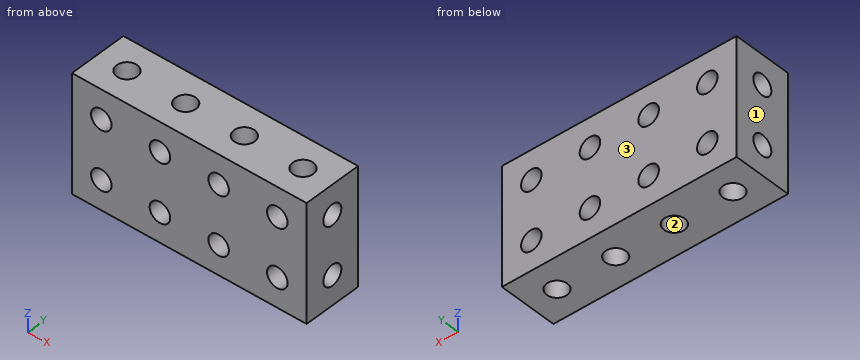
from build123d import *

# Parameters (mm, degrees)
ESQUISSE1_W             = 20
ESQUISSE1_H             = 10
BOSS_EXTRU_1_DEPTH      = 40
ESQUISSE2_R             = 1.75
ENL_V_MAT_EXTRU_1_DEPTH = 46.82575695
ESQUISSE3_R             = 1.75
ENL_V_MAT_EXTRU_2_DEPTH = 40
ESQUISSE4_R             = 1.75
ENL_V_MAT_EXTRU_3_DEPTH = 40


with BuildPart() as part:
    # Esquisse1 → Boss.-Extru.1 (new body)
    with BuildSketch(Plane(origin=(0, 0, 0), x_dir=(0, 0, -1), z_dir=(1, 0, 0))):
        with Locations((10, 5)):
            Rectangle(ESQUISSE1_W, ESQUISSE1_H)
    extrude(amount=BOSS_EXTRU_1_DEPTH)

    # Esquisse2 → Enlèv. mat.-Extru.1 (cut, through all)
    with BuildSketch(Plane(origin=(0, 10, 0), x_dir=(1, 0, 0), z_dir=(0, 1, 0))):
        with Locations(Location((5, 15, 0), (0, 0, 270))):
            Circle(ESQUISSE2_R)
        with Locations(Location((15, 15, 0), (0, 0, 270))):
            Circle(ESQUISSE2_R)
        with Locations(Location((25, 15, 0), (0, 0, 270))):
            Circle(ESQUISSE2_R)
        with Locations(Location((35, 15, 0), (0, 0, 270))):
            Circle(ESQUISSE2_R)
        with Locations(Location((5, 5, 0), (0, 0, 270))):
            Circle(ESQUISSE2_R)
        with Locations(Location((15, 5, 0), (0, 0, 270))):
            Circle(ESQUISSE2_R)
        with Locations(Location((25, 5, 0), (0, 0, 270))):
            Circle(ESQUISSE2_R)
        with Locations(Location((35, 5, 0), (0, 0, 270))):
            Circle(ESQUISSE2_R)
        with Locations((5, -5)):
            Circle(ESQUISSE2_R)
        with Locations((15, -5)):
            Circle(ESQUISSE2_R)
        with Locations((25, -5)):
            Circle(ESQUISSE2_R)
        with Locations((35, -5)):
            Circle(ESQUISSE2_R)
        with Locations((5, -15)):
            Circle(ESQUISSE2_R)
        with Locations((15, -15)):
            Circle(ESQUISSE2_R)
        with Locations((25, -15)):
            Circle(ESQUISSE2_R)
        with Locations((35, -15)):
            Circle(ESQUISSE2_R)
    extrude(amount=-ENL_V_MAT_EXTRU_1_DEPTH, mode=Mode.SUBTRACT)

    # Esquisse3 → Enlèv. mat.-Extru.2 (cut)
    with BuildSketch(Plane.XY):
        with Locations((5, 5)):
            Circle(ESQUISSE3_R)
        with Locations((15, 5)):
            Circle(ESQUISSE3_R)
        with Locations((25, 5)):
            Circle(ESQUISSE3_R)
        with Locations((35, 5)):
            Circle(ESQUISSE3_R)
    extrude(amount=-ENL_V_MAT_EXTRU_2_DEPTH, mode=Mode.SUBTRACT)

    # Esquisse4 → Enlèv. mat.-Extru.3 (cut)
    with BuildSketch(Plane(origin=(40, 0, 0), x_dir=(0, 0, -1), z_dir=(1, 0, 0))):
        with Locations((5, 5)):
            Circle(ESQUISSE4_R)
        with Locations(Location((15, 5, 0), (0, 0, 315))):
            Circle(ESQUISSE4_R)
        with Locations((25, 5)):
            Circle(ESQUISSE4_R)
        with Locations((35, 5)):
            Circle(ESQUISSE4_R)
    extrude(amount=-ENL_V_MAT_EXTRU_3_DEPTH, mode=Mode.SUBTRACT)


solid = part.part
The listing builds one solid part. Answer for the finished solid, in the listing's coordinates (mm). Face numbers are marked on the shaded views. Coordinates: 2 decimals unless noted, no trailing zeros. Write each loop counter-clockwise with the first axis right and the second up, starting at its lowest first coordinate (ties: lowest second). Pieces come first, ordered by that corner, then holes. Notation, with made-up numbers: M 48.5,11 L 90.5,11 A24 cw 90.5,25 Z; hole C 78.5,18 d3. An arc over 180 degrees is marked long. Write each question's results on one line, items separated by ' | '.
Item 1: The part is cut by section B-B on y = 8.75. State how many separate pieces and enclosed holes the cut face has, and give its area (3 significant figures).
Answer below:
separate pieces: 1 | enclosed holes: 8 | area: 723 mm2
Item 2: Consider probe 1 along X at (y, z) = (5, -9); probe 2 along Z at (x, y) = (12.5, 5); probe 3 along Z at (x, y) = (23, 6.25). Determine where each line is inside the solid, lowest interval first. Write a range as [from, to].
Answer below:
probe 1: [0, 3.25], [6.75, 13.25], [16.75, 23.25], [26.75, 33.25], [36.75, 40] | probe 2: [-20, -16.75], [-13.25, -6.75], [-3.25, 0] | probe 3: [-20, -16.22], [-13.78, -6.22], [-3.78, 0]
Item 3: The part is cut by section D-D on x = 8.5. Determine the outline of the cut face in (y, z), and give its area (3 significant figures).
Answer below:
outline: M 0,-20 L 10,-20 L 10,0 L 0,0 Z; hole C 5,-15 d3.5; hole C 5,-5 d3.5 | area: 181 mm2
Item 4: For a pull along X with two mould halves and no side action, classify the marked faces 1, 2 and 3 as released by +X, released by -X, zero draft, split by the parting line, or undercut.
Answer below:
face 1: released by -X | face 2: undercut | face 3: zero draft
Item 5: The part is cut by section A-A on x = 15. Determine the outline of the cut face in (y, z), and give its area (3 significant figures).
Answer below:
outline: M 0,-20 L 3.25,-20 L 3.25,-16.75 L 0,-16.75 Z; M 0,-13.25 L 3.25,-13.25 L 3.25,-6.75 L 0,-6.75 Z; M 0,-3.25 L 3.25,-3.25 L 3.25,0 L 0,0 Z; M 6.75,-20 L 10,-20 L 10,-16.75 L 6.75,-16.75 Z; M 6.75,-13.25 L 10,-13.25 L 10,-6.75 L 6.75,-6.75 Z; M 6.75,-3.25 L 10,-3.25 L 10,0 L 6.75,0 Z | area: 84.5 mm2
Item 6: The part is cut by section C-C on z = -1.5. Determine the outline of the cut face in (x, y), and give its area (3 significant figures).
Answer below:
outline: M 0,0 L 40,0 L 40,10 L 0,10 Z; hole C 5,5 d3.5; hole C 15,5 d3.5; hole C 25,5 d3.5; hole C 35,5 d3.5 | area: 362 mm2
